Part model, mm, in its own coordinate system. A direction names the side the tool comes from. Round coordinates to 2 decimals unless told otherwise and drop trailing zeros. Order: outer loops, then holes, each group sorted by start corner. A loop starts at its lowest first (then second) coordinate and runs counter-clockwise, first axis right, second up. Notation, with made-up numbers: (-3, 84.5) - (46, 84.5) arc R22 cw to (46, 114.5) - close; hole circle Ø7 at (-32.75, 27.25). An arc over 180 degrees is marked (long way). Return JSON: item names as keys, results as strings. Group by question number.
Item 1: Saw through at D-D on z = 164. List the corners of the cut face in (x, y), and give its area (3 significant figures).
Item 2: Tool access for faces 1 (the face through (150, 103, 180)), 2 (the face through (2.1, 50.14, 90.64)): list every direction of +Z, -Z, +X, -X, +Y, -Y with a clear straight run to the whole face (end or side of a thin tool).
Item 3: Two-plate mould, pull along Z, no slides. Class faces 3 (the face through (2.1, 43.34, 334.99)), 4 (the face through (2.1, 109.806, 233.674)), 5 (the face through (-150, 103, 180)), 6 (the face through (2.1, 50.62, 338.81)): released by +Z, released by -Z, zero draft, split by the parting line, or undercut.
Item 4: Saw through at B-B on x = 28. List the corners of the cut face in (y, z).
Item 5: Saw through at C-C on z = 263. List the corners of the cut face in (x, y).
Item 6: Probe probe 1 along Z at (x, y) = (57.5, 85); probe 2 along Z at (x, y) = (16, 61.5); probe 3 along Y at (x, z) = (-13.5, 73). List the from-to ranges inside material, lowest first.
Item 7: Saw through at A-A on y = 36.5. List the corners of the cut face in (x, z).
Item 8: Drop flat-ended pins along their axis: pin 1 (12 mm diameter, centred on x = 22.5, y = 56.5, fed in from +Z); pin 2 (1.5 mm diameter, centred on x = 116.5, y = 98, fed in from +Z); pin 3 (3 mm diameter, centred on x = 31.5, y = 66, fed in from -Z). Give the stop position or say it passes through.
```python
from build123d import *

# Parameters (mm, degrees)
BASE_FLANGE1_DEPTH = 150
FILLET_2_0_R       = 2


# Sheet-metal steps are written as plain solids
with BuildPart() as part:
    # Sketch1 → Base-Flange1 (new, symmetric)
    with BuildSketch(Plane(origin=(0, 0, 0), x_dir=(0, 0, -1), z_dir=(1, 0, 0))):
        with BuildLine():
            Line((-385, 0), (-283.559185115, 87.915372901))
            ThreePointArc((-283.559185115, 87.915372901), (-232.892960746, 109.891059496), (-178.771928145, 98.895109186))
            Line((-178.771928145, 98.895109186), (0, 0))
            Line((0, 0), (3.872491081, 7.000272339))
            Line((3.872491081, 7.000272339), (-174.899437063, 105.895381526))
            ThreePointArc((-174.899437063, 105.895381526), (-233.726646413, 117.847501428), (-288.798629422, 93.960885563))
            Line((-288.798629422, 93.960885563), (-390.239444307, 6.045512662))
            Line((-390.239444307, 6.045512662), (-385, 0))
        make_face()
    extrude(amount=BASE_FLANGE1_DEPTH, both=True)

    # Fillet-2.0
    fillet_2_0_edges = [part.edges().sort_by_distance(p)[0] for p in [
        (150, 3.022756331, 387.619722154),
        (150, 3.50013617, -1.936245541),
        (-150, 3.022756331, 387.619722154),
        (-150, 3.50013617, -1.936245541),
    ]]
    fillet(fillet_2_0_edges, radius=FILLET_2_0_R)


solid = part.part
```
Filled in:
{
 "1": {"outline": "(-150, 90.72) - (150, 90.72) - (150, 99.87) - (-150, 99.87) - close", "area": "2,740 mm^2"},
 "2": {"face 1": "+Z, -Z, +X, +Y, -Y", "face 2": "+X, -X, -Y"},
 "3": {"face 3": "undercut", "face 4": "undercut", "face 5": "zero draft", "face 6": "released by +Z"},
 "4": {"outline": "(0, 0) - (7, -3.87) - (105.9, 174.9) arc R100 ccw to (93.96, 288.8) - (6.05, 390.24) - (0, 385) - (87.92, 283.56) arc R92 cw to (98.9, 178.77) - close"},
 "5": {"outline": "(-150, 101.39) - (150, 101.39) - (150, 110.18) - (-150, 110.18) - close"},
 "6": {"probe 1": "z = 137.13 to 153.65, 286.92 to 299.14", "probe 2": "z = 94.65 to 111.17, 314.04 to 326.25", "probe 3": "y = 40.38 to 49.53"},
 "7": {"outline": "(-150, 49.45) - (150, 49.45) - (150, 65.98) - (-150, 65.98) - close; (-150, 342.88) - (150, 342.88) - (150, 355.1) - (-150, 355.1) - close"},
 "8": {"pin 1": "stops at z = 338.95", "pin 2": "stops at z = 284.8", "pin 3": "stops at z = 100.07"}
}
